The figure shows three views and two pictorial views of one solid part (mm, origin at its lowest corner). Answer the questions. A direction names the side the tool comes from. Coordinates: 2 decimals unless noted, no trailing zeros. Write each loop counter-clockwise with the first axis right and the second up, starting at its lowest first coordinate (ties: lowest second). Pieces come first, ordered by that corner, then holes.
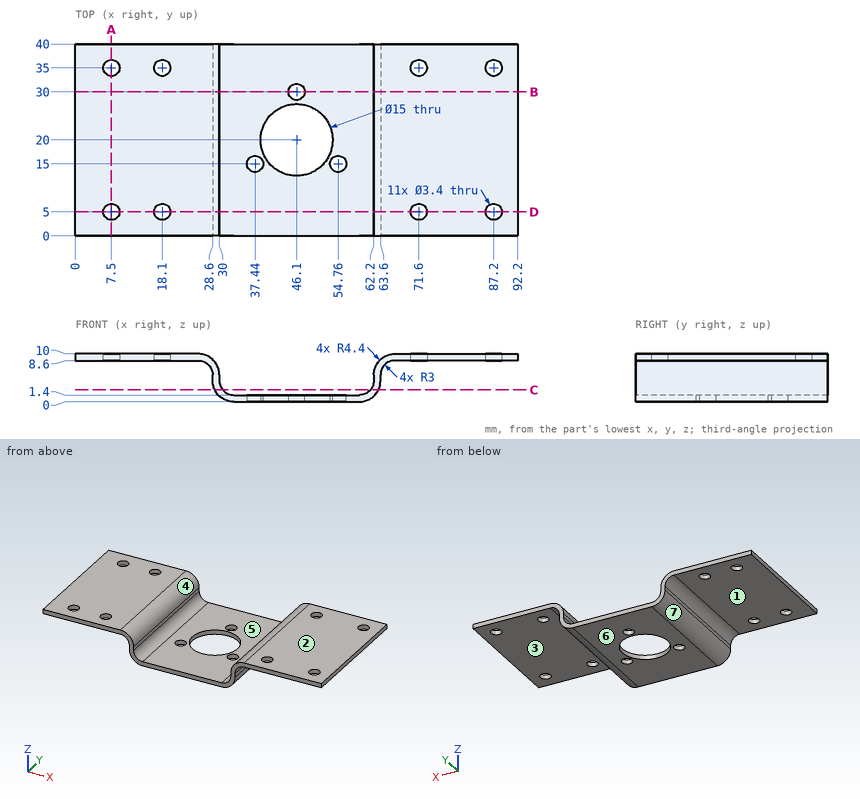
1. For a pull along X with two mould halves and no side action, classify the marked faces 4, 5, 6 and 7 as pulls with the +X half, pulls with the -X half, needs draft (parallel to the pull), parting line crosses it, or undercut.
Results found:
face 4: undercut
face 5: undercut
face 6: needs draft
face 7: pulls with the -X half
2. Flat-ended cylindrical pins translate along their axes: P1, Ø4, axis at y = 25.5, z = 9, coming from the -X side; P2, Ø8, axis at x = 56.5, y = 4.5, coming from the +Z side; P3, Ø8, axis at x = 19.5, y = 8, coming from the -Z side; P4, Ø4, axis at x = 83, z = 5, coming from the +Y side. Find the tip coordinate at first contact, or state that the pin passes through.
Results found:
P1: stops at x = 0
P2: stops at z = 1.7
P3: stops at z = 8.6
P4: passes through
3. Find the intervals of material crossed by L1, parallel to Y at x = 7.5, z = 9.45; L2, parallel to Y at x = 46.1, z = 0.75; L3, parallel to X at y = 16.5, z = 0.5 (1 decimal), in increasing order.
Results found:
L1: y = 0 to 3.3, 6.7 to 33.3, 36.7 to 40
L2: y = 0 to 12.5, 27.5 to 28.3, 31.7 to 40
L3: x = 31 to 36.6, 38.2 to 39.5, 52.7 to 54, 55.6 to 61.2
4. Section B-B on y = 30 is taken. Give the vertices of the cut face in (x, z).
Results found:
outline: (0, 8.6) - (25.6, 8.6) arc R3 cw to (28.6, 5.6) - (28.6, 4.4) arc R4.4 ccw to (33, 0) - (44.4, 0) - (44.4, 1.4) - (33, 1.4) arc R3 cw to (30, 4.4) - (30, 5.6) arc R4.4 ccw to (25.6, 10) - (0, 10) - close; (47.8, 0) - (59.2, 0) arc R4.4 ccw to (63.6, 4.4) - (63.6, 5.6) arc R3 cw to (66.6, 8.6) - (92.2, 8.6) - (92.2, 10) - (66.6, 10) arc R4.4 ccw to (62.2, 5.6) - (62.2, 4.4) arc R3 cw to (59.2, 1.4) - (47.8, 1.4) - close
5. Section A-A on x = 7.5 is taken. Give the vertices of the cut face in (y, z).
Results found:
outline: (0, 8.6) - (3.3, 8.6) - (3.3, 10) - (0, 10) - close; (6.7, 8.6) - (33.3, 8.6) - (33.3, 10) - (6.7, 10) - close; (36.7, 8.6) - (40, 8.6) - (40, 10) - (36.7, 10) - close
6. A tool of negligible diameter and unlimited length cuts with its end or side. For the marked faces 1, 2 and 3, from which of +Z, -Z, +X, -X, +Y, -Y can it reach the whole face along a straight path? Write none if from no direction.
Results found:
face 1: -Z, -X, +Y, -Y
face 2: +Z, +X, -X, +Y, -Y
face 3: -Z, +X, +Y, -Y
7. Section C-C on z = 2.5 is taken. Give the vertices of the cut face in (x, y), then the cut area to 3 significant figures.
Results found:
outline: (29.03, 0) - (30.68, 0) - (30.68, 40) - (29.03, 40) - close; (61.52, 0) - (63.17, 0) - (63.17, 40) - (61.52, 40) - close
area: 132 mm2
8. Section D-D on y = 5 is taken. State how many separate pieces and enclosed holes the cut face has, then the cut area to 3 significant figures.
Results found:
separate pieces: 5
enclosed holes: 0
area: 125 mm2
